Autodesk Inventor part; units mm, degrees
ref_plane "YZ Plane" through (0, 0, 0) normal (1, 0, 0) x (0, 1, 0)
ref_plane "XZ Plane" through (0, 0, 0) normal (0, 1, 0) x (-1, 0, 0)
sketch "Skizze1" plane through (0, 0, 0) normal (0, 1, 0) x (-1, 0, 0)
  line L0 (0, -5.01) -> (0, 6.96)
  line L1 (-0.7, 0) -> (-0.915, 0)
  line L2 (-0.915, 0) -> (-0.915, 0.41)
  line L3 (-0.915, 0.41) -> (-0.75, 0.41)
  line L4 (-0.75, 0.41) -> (-0.75, 3.99)
  line L5 (-0.75, 3.99) -> (-0.535, 3.99)
  line L6 (-0.535, 3.99) -> (-0.535, 6.425)
  arc A0 (0, 6.96) -> (-0.535, 6.425) centre (0, 6.425) ccw
  line L7 (-0.535, 6.425) -> (0, 6.425) construction
  line L8 (-0.7, 0) -> (-0.7, -0.71)
  line L9 (-0.7, -0.71) -> (-0.32, -0.71)
  line L10 (-0.32, -0.71) -> (-0.32, -5.01)
  line L11 (-0.32, -5.01) -> (0, -5.01)
  line L12 (0, -7.4262) -> (0, 9.487)
  line L13 (-1.098, 0) -> (0.183, 0)
  dimension "d0" = 1.07
  dimension "d1" = 0.41
  dimension "d2" = 1.83
  dimension "d3" = 1.5
  dimension "d5" = 6.96
  dimension "d10" = 0.71
  dimension "d11" = 0.7
  dimension "d12" = 4.3
  dimension "d15" = 0.64
  dimension "d16" = 4.7
revolve "Umdrehung1" add sketch "Skizze1" angle 360 about axis through (0, 0, -5.01) along (0, 0, 1)
chamfer "Fase1" distance 0.1 angle 45 1 edges at (-0.75, 0, 3.99)
ref_plane "Arbeitsebene2" through (0, 0, 4.67) normal (0, 0, 1) x (1, 0, 0)
ref_plane "Arbeitsebene1" through (0, 0, 6.96) normal (0, 0, 1) x (1, 0, 0)
properties part number "Federkontakt D1.5" material "Kupfer, Legierung"
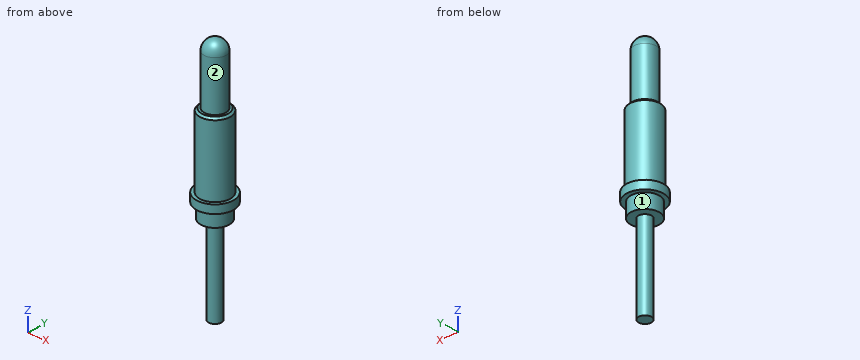
Could you check a few things on this model? Use its own coordinates, in mm. Face numbers are marked on the shaded views. A direction names the side the tool comes from. Coordinates: 2 decimals unless noted, no trailing zeros. Write each loop counter-clockwise with the first axis right and the second up, starting at its lowest first coordinate (ties: lowest second). Pieces come first, ordered by that corner, then holes. Notation, with made-up numbers: (37, 40) -> (66, 40) arc R27 cw to (66, 67) -> close; hole circle Ø6 at (50, 71). An arc over 180 degrees is marked (long way). Return JSON: item names as keys, results as strings.
(1) I need wall thicknesses on L1, parallel to Z at x = -0.3, y = 0.8; L2, parallel to Y at x = 0, z = 0.5; L3, parallel to X at y = 0.15, z = -4. Which ranges of each line are inside material? Lowest first, please.
Numbers:
{"L1": "z = 0 to 0.41", "L2": "y = -0.75 to 0.75", "L3": "x = -0.28 to 0.28"}
(2) Imagine slicing it at A-A, the plane x = 0. Please give me the cut outline in (y, z) (3 decimals), then the cut area to 3 significant figures.
Numbers:
{"outline": "(-0.915, 0) -> (-0.7, 0) -> (-0.7, -0.71) -> (-0.32, -0.71) -> (-0.32, -5.01) -> (0.32, -5.01) -> (0.32, -0.71) -> (0.7, -0.71) -> (0.7, 0) -> (0.915, 0) -> (0.915, 0.41) -> (0.75, 0.41) -> (0.75, 3.89) -> (0.65, 3.99) -> (0.535, 3.99) -> (0.535, 6.425) arc R0.535 ccw to (-0.535, 6.425) -> (-0.535, 3.99) -> (-0.65, 3.99) -> (-0.75, 3.89) -> (-0.75, 0.41) -> (-0.915, 0.41) -> close", "area": "12.9 mm2"}
(3) Imagine slicing it at C-C, the plane z = 3.5. Please give me the cut outline in (x, y).
Numbers:
{"outline": "circle Ø1.5 at (0, 0)"}
(4) Imagine slicing it at D-D, the plane z = -1. Please give me the cut outline in (x, y), then the cut area to 3 significant figures.
Numbers:
{"outline": "circle Ø0.64 at (0, 0)", "area": "0.322 mm2"}
(5) Which directions (+Z, -Z, +X, -X, +Y, -Y) give clear straight access to the entire face, cutting with the end or side of a thin tool? Please do the marked faces 1 and 2.
Numbers:
{"face 1": "-Z", "face 2": "+Z"}
(6) I'm going to push a flat-ended pin straight in: pin 1 (1 mm diameter, centred on x = -0.5, y = -0.5, fed in from +Z). Where does the tip first touch, or does it pass through?
Numbers:
{"pin 1": "stops at z = 6.92"}
